Autodesk Inventor part; units mm, degrees
ref_plane "YZ Plane" through (0, 0, 0) normal (1, 0, 0) x (0, 1, 0)
ref_plane "XZ Plane" through (0, 0, 0) normal (0, 1, 0) x (-1, 0, 0)
ref_plane "XY Plane" through (0, 0, 0) normal (0, 0, 1) x (1, 0, 0)
sketch "Sketch1" plane through (0, 0, 0) normal (0, 1, 0) x (-1, 0, 0)
  point P0 (0, 0)
sketch "Sketch2" plane through (0, 0, 0) normal (0, 1, 0) x (-1, 0, 0)
  line L0 (0, 0) -> (1320.8, 0)
  line L1 (1320.8, 0) -> (1320.8, 698.5)
  line L2 (1320.8, 698.5) -> (0, 698.5)
  line L3 (0, 698.5) -> (0, 0)
  dimension "d0" = 1320.8
  dimension "d1" = 698.5
extrude "Extrusion1" add sketch "Sketch2" along normal blind 762
shell "Shell1" thickness 2.54 removed faces 1 at (-440.2667, 762, 465.6667)
properties part number "Crate Stacker"
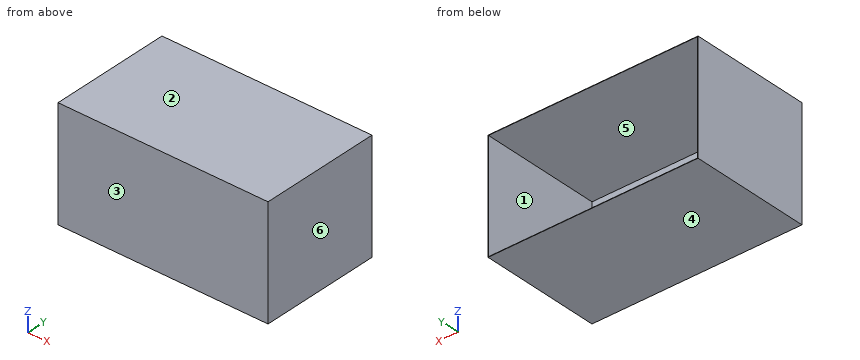
Work out the finished part from the listing and answer in its coordinate system (mm). Face numbers are marked on the shaded views. A direction names the side the tool comes from. Give positions to 0.01 mm unless a question says otherwise; leave off trailing zeros. Order: outer loops, then holes, each group sorted by start corner. A loop starts at its lowest first (then second) coordinate and runs counter-clockwise, first axis right, second up. Notation, with made-up numbers: (67, -9) -> (96, -9) arc R14 ccw to (96, -3) -> close; hole circle Ø9 at (-29, 12.5). An arc over 180 degrees is marked (long way). Answer as CSV lines item,"result". Start each with the question number.
(1) Section B-B, the plane x = -906 is taken. Write down the section's boundary in (y, z).
(2) Which of the six approach directions +Z, -Z, +X, -X, +Y, -Y give full straight-line access (tool end or side, diameter ignored) to the marked faces 5 and 6?
(3) Consider line 1 along X through (y, z) = (83, 381); line 2 along Z through (x, y) = (-795.5, 117); line 3 along Y through (x, z) = (-699, 375.5). Determine where each line is inside the solid, lowest interval first.
(4) For a pull along Z with two mould halves and no side action, classify the marked faces 1, 2, 3 and 4 as released by +Z, released by -Z, zero draft, split by the parting line, or undercut.
(5) This flat-tipped pin is pushed along its axis until it touches: pin 1 Ø2 at (x, z) = (-687.5, 149.5) entering from +Y. Where does it stop, or does it pass through?
(6) Section C-C, the plane z = 158.5 is taken. Write down the section's boundary in (x, y).
(7) Section A-A, the plane y = 410.5 is taken. Write down the section's boundary in (x, z).
Entries:
1,outline,"(0, 0) -> (762, 0) -> (762, 2.54) -> (2.54, 2.54) -> (2.54, 695.96) -> (762, 695.96) -> (762, 698.5) -> (0, 698.5) -> close"
2,face 5,"+Y"
2,face 6,"+Z, -Z, +X, +Y, -Y"
3,line 1,"-1320.8 to -1318.26, -2.54 to 0"
3,line 2,"0 to 2.54, 695.96 to 698.5"
3,line 3,"0 to 2.54"
4,face 1,"undercut"
4,face 2,"released by +Z"
4,face 3,"zero draft"
4,face 4,"released by -Z"
5,pin 1,"y = 2.54"
6,outline,"(-1320.8, 0) -> (0, 0) -> (0, 762) -> (-2.54, 762) -> (-2.54, 2.54) -> (-1318.26, 2.54) -> (-1318.26, 762) -> (-1320.8, 762) -> close"
7,outline,"(-1320.8, 0) -> (0, 0) -> (0, 698.5) -> (-1320.8, 698.5) -> close; hole (-1318.26, 2.54) -> (-2.54, 2.54) -> (-2.54, 695.96) -> (-1318.26, 695.96) -> close"
